```python
from build123d import *

# Parameters (mm, degrees)
BOSS_EXTRUDE1_DEPTH       = 20
M3_CLEARANCE_SLOT1_DEPTH  = 8.2
SKETCH5_W                 = 3.2
SKETCH5_H                 = 9.75
CUT_EXTRUDE1_DEPTH        = 37.976208567
CUT_EXTRUDE2_DEPTH        = 37.400549446
LPATTERN1_COUNT           = 2
LPATTERN1_PITCH           = 10
LPATTERN2_COUNT           = 2
LPATTERN2_PITCH           = 10
FILLET2_R                 = 0.5
SKETCH9_W                 = 2
SKETCH9_H                 = 20
BOSS_EXTRUDE2_DEPTH       = 1.35
FILLET1_R                 = 1
M2X0_4_TAPPED_HOLE1_D     = 1.6
M2X0_4_TAPPED_HOLE1_DEPTH = 2


# Read off the part's stored shape, not the designer's step: M3 Clearance Slot1
with BuildPart() as part:
    # Sketch2 → Boss-Extrude1 (new body)
    with BuildSketch(Plane(origin=(0, 0, 0), x_dir=(1, 0, 0), z_dir=(0, 1, 0))):
        Polygon((0, -30), (0, 30), (8.2, 30), (8.2, 16.25), (6.2, 16.25), (6.2, 17.75), (5, 17.75), (5, -17.75), (6.2, -17.75), (6.2, -16.25), (8.2, -16.25), (8.2, -30), align=None)
    extrude(amount=BOSS_EXTRUDE1_DEPTH)

    # M3 Clearance Slot1 outline → M3 Clearance Slot1 (cut)
    with BuildSketch(Plane.YZ):
        with BuildLine():
            ThreePointArc((15.8, 22.4), (17.5, 24.1), (15.8, 25.8))
            Line((15.8, 25.8), (4.2, 25.8))
            ThreePointArc((4.2, 25.8), (2.5, 24.1), (4.2, 22.4))
            Line((4.2, 22.4), (15.8, 22.4))
        make_face()
        with BuildLine():
            ThreePointArc((15.8, -25.8), (17.5, -24.1), (15.8, -22.4))
            Line((15.8, -22.4), (4.2, -22.4))
            ThreePointArc((4.2, -22.4), (2.5, -24.1), (4.2, -25.8))
            Line((4.2, -25.8), (15.8, -25.8))
        make_face()
    extrude(amount=M3_CLEARANCE_SLOT1_DEPTH, mode=Mode.SUBTRACT)

    # Sketch5 → Cut-Extrude1 (cut, through all)
    with BuildSketch(Plane.XZ):
        with Locations((6.6, 25.125)):
            Rectangle(SKETCH5_W, SKETCH5_H)
        with Locations((6.6, -25.125)):
            Rectangle(SKETCH5_W, SKETCH5_H)
    extrude(amount=-CUT_EXTRUDE1_DEPTH, mode=Mode.SUBTRACT)

    # Sketch8 → Cut-Extrude2 (cut, through all)
    with BuildSketch(Plane(origin=(5, 0, 0), x_dir=(0, 0, -1), z_dir=(1, 0, 0))):
        Polygon((0, 5), (2.886751346, 10), (0, 15), (-2.886751346, 10), align=None)
    cut_extrude2 = extrude(amount=-CUT_EXTRUDE2_DEPTH, mode=Mode.SUBTRACT)

    # LPattern1: Cut-Extrude2 ×2
    with Locations(*[(0, 0, i * LPATTERN1_PITCH) for i in range(1, LPATTERN1_COUNT)]):
        add(cut_extrude2, mode=Mode.SUBTRACT)

    # LPattern2: Cut-Extrude2 ×2
    with Locations(*[(0, 0, -i * LPATTERN2_PITCH) for i in range(1, LPATTERN2_COUNT)]):
        add(cut_extrude2, mode=Mode.SUBTRACT)

    # Fillet2
    fillet2_edges = [part.edges().sort_by_distance(p)[0] for p in [
        (5, 10, 20.25),
        (5, 10, -20.25),
    ]]
    fillet(fillet2_edges, radius=FILLET2_R)

    # Sketch9 → Boss-Extrude2 (add)
    with BuildSketch(Plane.XY.offset(-16.25)):
        with Locations((7.2, 10)):
            Rectangle(SKETCH9_W, SKETCH9_H)
    extrude(amount=BOSS_EXTRUDE2_DEPTH)

    # Fillet1
    fillet1_edges = [part.edges().sort_by_distance(p)[0] for p in [
        (8.2, 10, 16.25),
        (8.2, 10, 20.25),
        (5, 10, 30),
        (8.2, 10, -20.25),
        (5, 10, -30),
    ]]
    fillet(fillet1_edges, radius=FILLET1_R)

    # M2x0.4 Tapped Hole1
    with Locations(Plane(origin=(8.2, 0, 0), x_dir=(0, 0, -1), z_dir=(1, 0, 0))):
        with Locations((16.5, 10)):
            Hole(M2X0_4_TAPPED_HOLE1_D / 2, depth=M2X0_4_TAPPED_HOLE1_DEPTH)


solid = part.part
```
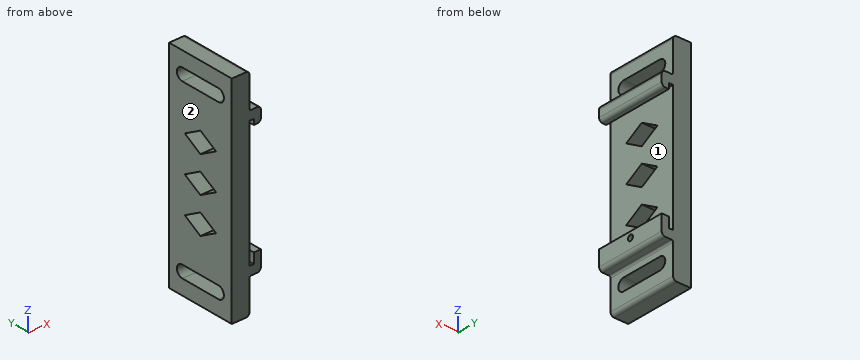
The model under review builds one solid part; all positions refer to its coordinate system, in mm. Face numbers are marked on the shaded views. Round coordinates to 2 decimals unless told otherwise and drop trailing zeros. Loops run counter-clockwise (first coordinate to the right, second up) from the corner with the lowest first, then second, coordinate; pieces in that order, holes last. Notation, with made-up numbers: (3, -15.5) - (40, -15.5) arc R17 ccw to (40, 17.5) - close; hole circle Ø1 at (-20, 10). An arc over 180 degrees is marked (long way). Use a Markdown table: item, result. Add a question column.
Q1. Add section B-B (x = 1.5). State the section outline as (y, z) points.
Q2. Insertion check: pin 1 Ø0.8 at (y, z) = (8, 17) entering from -X; pin 2 Ø0.8 at (x, y) = (6.5, 9.5) entering from -Z; pin 3 Ø3 at (y, z) = (12.5, -23) entering from +X; pin 4 Ø1 at (x, y) = (7.5, 12.5) entering from +Z. Each pin has a flat end and moves straight along its axis. Give the tip position at first contact, or say it passes through.
Q3. Add section C-C (z = -24.1). State the section outline as (x, y) points, plus the area to 3 significant figures.
Q4. Add section D-D (y = 7). State how many separate pieces and enclosed holes the cut face has, plus the area to 3 significant figures.
Q5. For probe 1 along Y at (x, z) = (6.8, -16.5); probe 2 along Z at (x, y) = (0.75, 9.5); probe 3 along Z at (x, y) = (7.25, 12.75), list the stretches that pass through material, from the lowest coordinate up.
Q6. The part is to be moulded in two halves that separate along Z. For the marked faces 1 and 2, say which applies: pulls with the +Z half, pulls with the -Z half, needs draft (parallel to the pull), parting line crosses it, or undercut.
Q7. Add section A-A (z = -16.5). State the section outline as (x, y) points.
Worked answers:
| question | item | result |
|---|---|---|
| 1 | outline | (0, -30) - (20, -30) - (20, 30) - (0, 30) - close; hole (4.2, -25.8) - (15.8, -25.8) arc R1.7 ccw to (15.8, -22.4) - (4.2, -22.4) arc R1.7 ccw to start; hole (4.2, 22.4) - (15.8, 22.4) arc R1.7 ccw to (15.8, 25.8) - (4.2, 25.8) arc R1.7 ccw to start; hole (5, -10) - (10, -12.89) - (15, -10) - (10, -7.11) - close; hole (5, 0) - (10, -2.89) - (15, 0) - (10, 2.89) - close; hole (5, 10) - (10, 7.11) - (15, 10) - (10, 12.89) - close |
| 2 | pin 1 | x = 0 |
| 2 | pin 2 | z = -20.25 |
| 2 | pin 3 | x = 5 |
| 2 | pin 4 | z = 20.25 |
| 3 | outline | (0, 0) - (5, 0) - (5, 2.5) - (0, 2.5) - close; (0, 17.5) - (5, 17.5) - (5, 20) - (0, 20) - close |
| 3 | area | 25.0 mm² |
| 4 | separate pieces | 6 |
| 4 | enclosed holes | 0 |
| 4 | area | 255 mm² |
| 5 | probe 1 | 0 to 9.2, 10.8 to 20 |
| 5 | probe 2 | -30 to -25.8, -22.4 to -12.6, -7.4 to -2.6, 2.6 to 7.4, 12.6 to 22.4, 25.8 to 30 |
| 5 | probe 3 | -20.25 to -14.9, 16.25 to 20.25 |
| 6 | face 1 | undercut |
| 6 | face 2 | needs draft |
| 7 | outline | (0, 0) - (5, 0) - (5, 20) - (0, 20) - close; (6.2, 0) - (8.2, 0) - (8.2, 9.2) - (6.2, 9.2) - close; (6.2, 10.8) - (8.2, 10.8) - (8.2, 20) - (6.2, 20) - close |
